Input: part model. Units: mm. Frame: model coordinates. Give positions to 0.01 mm unless a question says otherwise; leave off trailing zeros. Loops run counter-clockwise (first coordinate to the right, second up) from the corner with the lowest first, then second, coordinate; pieces in that order, holes last. Notation, with made-up numbers: (-31.5, -32.5) -> (-24.5, -32.5) arc R21 ccw to (-24.5, 1.5) -> close; hole circle Ø5 at (5, 6.25). An arc over 180 degrees is marked (long way). Answer as a JSON object with one key per item and string values.
```python
from build123d import *

# Parameters (mm, degrees)
SKETCH1_R           = 0.75
BOSS_EXTRUDE1_DEPTH = 0.5


with BuildPart() as part:
    # Sketch1 → Boss-Extrude1 (new body)
    with BuildSketch(Plane(origin=(0, 0, 0), x_dir=(1, 0, 0), z_dir=(0, 1, 0))):
        with BuildLine():
            Line((-39.503518064, 27.177881063), (-43.503518064, 27.177881063))
            ThreePointArc((-43.503518064, 27.177881063), (-39.392691136, 22.257579116), (-33.819769565, 25.427881063))
            Line((-33.819769565, 25.427881063), (-31.753518064, 25.427881063))
            Line((-31.753518064, 25.427881063), (-31.753518064, 24.177881063))
            Line((-31.753518064, 24.177881063), (-30.503518064, 24.177881063))
            Line((-30.503518064, 24.177881063), (-30.503518064, 26.302881063))
            Line((-30.503518064, 26.302881063), (-30.503518064, 27.177881063))
            Line((-30.503518064, 27.177881063), (-37.503518064, 27.177881063))
            ThreePointArc((-37.503518064, 27.177881063), (-37.796411282, 26.470774282), (-38.503518064, 26.177881063))
            ThreePointArc((-38.503518064, 26.177881063), (-39.210624845, 26.470774282), (-39.503518064, 27.177881063))
        make_face()
        with BuildLine():
            ThreePointArc((-40.003518064, 24.177881063), (-39.564178235, 25.238541235), (-38.503518064, 25.677881063))
            ThreePointArc((-38.503518064, 25.677881063), (-37.442857892, 25.238541235), (-37.003518064, 24.177881063))
            ThreePointArc((-37.003518064, 24.177881063), (-38.503518064, 22.677881063), (-40.003518064, 24.177881063))
        make_face(mode=Mode.SUBTRACT)
        with Locations(Location((-41.253518064, 25.427881063, 0), (0, 0, 270))):
            Circle(SKETCH1_R, mode=Mode.SUBTRACT)
        with Locations(Location((-35.753518064, 25.427881063, 0), (0, 0, 270))):
            Circle(SKETCH1_R, mode=Mode.SUBTRACT)
        Polygon((-31.003518064, 26.802881063), (-31.003518064, 26.302881063), (-31.003518064, 25.802881063), (-33.003518064, 25.802881063), (-33.003518064, 26.802881063), align=None, mode=Mode.SUBTRACT)
    extrude(amount=BOSS_EXTRUDE1_DEPTH)


solid = part.part
```
Q1. Ray query, line 1 along X through (y, z) = (0.3, -24.95); line 2 along X through (y, z) = (0.35, -24.35); line 3 along Z through (x, y) = (-41.25, 0.45). Return the intervals inside material, ascending.
Evaluation:
{"line 1": "x = -42.98 to -41.83, -40.68 to -39.79, -37.22 to -36.33, -35.18 to -34.03, -31.75 to -30.5", "line 2": "x = -42.63 to -39.99, -37.01 to -34.38, -31.75 to -30.5", "line 3": "z = -27.18 to -26.18, -24.68 to -23"}
Q2. Section B-B, the plane z = -25.05. Return the cut outline in (x, y).
Evaluation:
{"outline": "(-43.03, 0) -> (-41.9, 0) -> (-41.9, 0.5) -> (-43.03, 0.5) -> close; (-40.61, 0) -> (-39.72, 0) -> (-39.72, 0.5) -> (-40.61, 0.5) -> close; (-37.28, 0) -> (-36.4, 0) -> (-36.4, 0.5) -> (-37.28, 0.5) -> close; (-35.11, 0) -> (-33.98, 0) -> (-33.98, 0.5) -> (-35.11, 0.5) -> close; (-31.75, 0) -> (-30.5, 0) -> (-30.5, 0.5) -> (-31.75, 0.5) -> close"}
Q3. Section A-A, the plane x = -32.25. Return the cut outline in (y, z).
Evaluation:
{"outline": "(0, -27.18) -> (0.5, -27.18) -> (0.5, -26.8) -> (0, -26.8) -> close; (0, -25.8) -> (0.5, -25.8) -> (0.5, -25.43) -> (0, -25.43) -> close"}
Q4. Section C-C, the plane z = -24.5. Return the cut outline in (x, y).
Evaluation:
{"outline": "(-42.73, 0) -> (-39.97, 0) -> (-39.97, 0.5) -> (-42.73, 0.5) -> close; (-37.04, 0) -> (-34.28, 0) -> (-34.28, 0.5) -> (-37.04, 0.5) -> close; (-31.75, 0) -> (-30.5, 0) -> (-30.5, 0.5) -> (-31.75, 0.5) -> close"}
Q5. Section D-D, the plane y = 0.3. Return the cut outline in (x, z), then the cut area to 3 significant figures.
Evaluation:
{"outline": "(-43.5, -27.18) -> (-39.5, -27.18) arc R1 cw to (-37.5, -27.18) -> (-30.5, -27.18) -> (-30.5, -24.18) -> (-31.75, -24.18) -> (-31.75, -25.43) -> (-33.82, -25.43) arc R5 ccw to start; hole circle Ø1.5 at (-41.25, -25.43); hole circle Ø3 at (-38.5, -24.18); hole circle Ø1.5 at (-35.75, -25.43); hole (-33, -26.8) -> (-31, -26.8) -> (-31, -25.8) -> (-33, -25.8) -> close", "area": "32.1 mm2"}
Q6. Draft query along X for faces 1 (the cylindrical face through (-41.92, 0.25, -25.08)), 2 (the flat face through (-37, 0, -25)). Return one class per face: +X half, -X half, draft (parallel to the pull), parting line (faces both ways), or undercut.
Evaluation:
{"face 1": "undercut", "face 2": "draft"}
